Can you work these out from the model? Positions are in its coordinate system, mm. Face numbers are marked on the shaded views. A direction names the side the tool comes from. Give positions to 0.01 mm unless a question says otherwise; leave off trailing zeros. Loops run counter-clockwise (first coordinate to the right, second up) from the corner with the lowest first, then second, coordinate; pieces in that order, holes last. Notation, with made-up numbers: (2.5, -11.5) - (47.5, -11.5) arc R10 cw to (47.5, 3.5) - close; hole circle Ø9 at (43, 68.25). An arc over 180 degrees is marked (long way). Answer as a JSON object with one key per item and string values. Group by question number.
Item 1: Please list where these lines run through material, in increasing order: L1, parallel to Y at x = -10, z = 21; L2, parallel to Y at x = -6.75, z = 6.25; L3, parallel to Z at x = -5.5, y = -6.
Item 2: Thinking about a two-plate mould opening in Y: for the marked faces 1, 2 and 3, which applies, pulls with the +Y half, pulls with the -Y half, needs draft (parallel to the pull), parting line crosses it, or undercut?
Item 3: Suppose I cut it at D-D on x = 10.5. Write out the boundary of the cut face in (y, z), and give its area (3 significant figures).
Item 4: Suppose I cut it at B-B on z = 4.5. Write out the boundary of the cut face in (x, y).
Item 5: Which directions (+Z, -Z, +X, -X, +Y, -Y) give clear straight access to the entire face, cutting with the end or side of a thin tool? Please do the marked faces 4 and 5.
Item 6: Suppose I cut it at C-C on x = 0. Write out the boundary of the cut face in (y, z).
Item 7: Suppose I cut it at A-A on y = 0. Write out the boundary of the cut face in (x, z), and give its area (3 significant figures).
Item 8: Will these pins go through, and if not, where does the flat tip stop? pin 1 (4 mm diameter, centred on y = 15, z = 21, fed in from +X); pin 2 (1.5 mm diameter, centred on x = 0, y = 18.5, fed in from -Z); pin 3 (5 mm diameter, centred on y = -15, z = 21, fed in from -X) (3 decimals); pin 4 (10 mm diameter, centred on x = 9, y = -4.5, fed in from -Z).
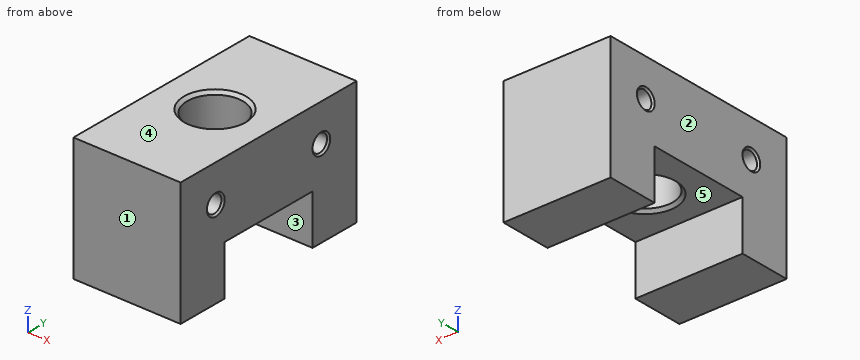
from build123d import *

# Parameters (mm, degrees)
SKETCH1_W                      = 26
SKETCH1_H                      = 50
BOSS_EXTRUDE1_DEPTH            = 30
SKETCH2_W                      = 26
SKETCH2_H                      = 25
CUT_EXTRUDE1_DEPTH             = 12
M5X0_8_TAPPED_HOLE1_AT_2_COUNT = 2
M5X0_8_TAPPED_HOLE1_AT_2_PITCH = 30


with BuildPart() as part:
    # Sketch1 → Boss-Extrude1 (new body)
    with BuildSketch(Plane.XY):
        Rectangle(SKETCH1_W, SKETCH1_H)
    extrude(amount=BOSS_EXTRUDE1_DEPTH)

    # Sketch2 → Cut-Extrude1 (cut)
    with BuildSketch(Plane.XY):
        Rectangle(SKETCH2_W, SKETCH2_H)
    extrude(amount=CUT_EXTRUDE1_DEPTH, mode=Mode.SUBTRACT)

    # Sketch8 → M12 Clearance Hole1 (revolve, cut)
    with BuildSketch(Plane(origin=(0, 0, 12), x_dir=(0, 1, 0), z_dir=(1, 0, 0))):
        Polygon((0, 0), (0, 18), (7.5, 18), (6.75, 17.25), (6.75, 0.75), (7.5, 0), align=None)
    revolve(axis=Axis((0, 0, 5.65), (0, 0, 1)), mode=Mode.SUBTRACT)

    # Sketch11 → M5x0.8 Tapped Hole1 (revolve, cut)
    with BuildSketch(Plane(origin=(13, 15, 21), x_dir=(0, 0, -1), z_dir=(0, 1, 0))):
        Polygon((0, 0), (0, 12), (2.1, 10.7381927), (2.1, 0.425), (2.525, 0), align=None)
    m5x0_8_tapped_hole1 = revolve(axis=Axis((19.35, 15, 21), (-1, 0, 0)), mode=Mode.SUBTRACT)

    # M5x0.8 Tapped Hole1 at 2: M5x0.8 Tapped Hole1 ×2
    with Locations(*[(0, -i * M5X0_8_TAPPED_HOLE1_AT_2_PITCH, 0) for i in range(1, M5X0_8_TAPPED_HOLE1_AT_2_COUNT)]):
        add(m5x0_8_tapped_hole1, mode=Mode.SUBTRACT)

    # Mirror1: M5x0.8 Tapped Hole1 across plane
    add(m5x0_8_tapped_hole1.mirror(Plane(origin=(0, 0, 0), x_dir=(0, 0, 1), z_dir=(1, 0, 0))), mode=Mode.SUBTRACT)

    # Mirror1 copy 1 sketch → Mirror1 copy 1 (revolve, cut)
    with BuildSketch(Plane(origin=(-13, -15, 21), x_dir=(0, 0, -1), z_dir=(0, 1, 0))):
        Polygon((0, 0), (0, -12), (2.1, -10.7381927), (2.1, -0.425), (2.525, 0), align=None)
    revolve(axis=Axis((-19.35, -15, 21), (-1, 0, 0)), mode=Mode.SUBTRACT)


solid = part.part
Worked out:
{
 "1": {"L1": "y = -25 to -17.1, -12.9 to 12.9, 17.1 to 25", "L2": "y = -25 to -12.5, 12.5 to 25", "L3": "z = 12 to 30"},
 "2": {"face 1": "pulls with the -Y half", "face 2": "needs draft", "face 3": "undercut"},
 "3": {"outline": "(-25, 0) - (-12.5, 0) - (-12.5, 12) - (12.5, 12) - (12.5, 0) - (25, 0) - (25, 30) - (-25, 30) - close; hole circle Ø4.2 at (-15, 21); hole circle Ø4.2 at (15, 21)", "area": "1,170 mm2"},
 "4": {"outline": "(-13, -25) - (13, -25) - (13, -12.5) - (-13, -12.5) - close; (-13, 12.5) - (13, 12.5) - (13, 25) - (-13, 25) - close"},
 "5": {"face 4": "+Z, +X, -X, +Y, -Y", "face 5": "-Z, +X, -X"},
 "6": {"outline": "(-25, 0) - (-12.5, 0) - (-12.5, 12) - (-7.5, 12) - (-6.75, 12.75) - (-6.75, 29.25) - (-7.5, 30) - (-25, 30) - close; (6.75, 12.75) - (7.5, 12) - (12.5, 12) - (12.5, 0) - (25, 0) - (25, 30) - (7.5, 30) - (6.75, 29.25) - close"},
 "7": {"outline": "(-13, 12) - (-7.5, 12) - (-6.75, 12.75) - (-6.75, 29.25) - (-7.5, 30) - (-13, 30) - close; (6.75, 12.75) - (7.5, 12) - (13, 12) - (13, 30) - (7.5, 30) - (6.75, 29.25) - close", "area": "224 mm2"},
 "8": {"pin 1": "stops at x = 2.2", "pin 2": "stops at z = 0", "pin 3": "stops at x = -12.975", "pin 4": "stops at z = 12"}
}
